from build123d import *

# Parameters (mm, degrees)
SKETCH1_R               = 19.05
BASE_EXTRUDE_DEPTH      = 47.625
CUT_EXTRUDE1_DEPTH      = 20.05
CUT_EXTRUDE1_DEPTH_BACK = 20.05
SKETCH8_W               = 20.32
SKETCH8_H               = 36.600526062
CUT_EXTRUDE5_DEPTH      = 47.625
CUT_EXTRUDE5_DEPTH_BACK = 20.0500001
SKETCH11_R              = 4.7625
CUT_EXTRUDE6_DEPTH      = 20.0500001
CUT_EXTRUDE6_DEPTH_BACK = 20.0500001
SKETCH12_R              = 6.35
BOSS_EXTRUDE1_DEPTH     = 19.05
CHAMFER3_SIZE           = 1.27
CHAMFER3_SIZE2          = 2.199704526
CUT_EXTRUDE7_DEPTH      = 12.7


with BuildPart() as part:
    # Sketch1 → Base-Extrude (new body)
    with BuildSketch(Plane(origin=(0, 0, 0), x_dir=(-1, 0, 0), z_dir=(0, 1, 0))):
        Circle(SKETCH1_R)
    extrude(amount=BASE_EXTRUDE_DEPTH)

    # Sketch2 → Cut-Extrude1 (cut, two sides)
    with BuildSketch(Plane.XY) as cut_extrude1_sk:
        with BuildLine():
            Line((9.525, 9.525), (9.525, 19.685))
            ThreePointArc((9.525, 19.685), (12.314807909, 26.420192091), (19.05, 29.21))
            Line((19.05, 29.21), (19.05, -1.366191125))
            Line((19.05, -1.366191125), (-19.05, -1.366191125))
            Line((-19.05, -1.366191125), (-19.05, 29.21))
            ThreePointArc((-19.05, 29.21), (-12.314807909, 26.420192091), (-9.525, 19.685))
            Line((-9.525, 19.685), (-9.525, 9.525))
            ThreePointArc((-9.525, 9.525), (0, 0), (9.525, 9.525))
        make_face()
    extrude(amount=CUT_EXTRUDE1_DEPTH, mode=Mode.SUBTRACT)
    extrude(cut_extrude1_sk.sketch, amount=-CUT_EXTRUDE1_DEPTH_BACK, mode=Mode.SUBTRACT)

    # Sketch8 → Cut-Extrude5 (cut, two sides)
    with BuildSketch(Plane(origin=(0, 0, 0), x_dir=(0, 0, -1), z_dir=(1, 0, 0))) as cut_extrude5_sk:
        with Locations((0, 10.844975795)):
            Rectangle(SKETCH8_W, SKETCH8_H)
    extrude(amount=CUT_EXTRUDE5_DEPTH, mode=Mode.SUBTRACT)
    extrude(cut_extrude5_sk.sketch, amount=-CUT_EXTRUDE5_DEPTH_BACK, mode=Mode.SUBTRACT)

    # Sketch11 → Cut-Extrude6 (cut, two sides)
    with BuildSketch(Plane.XY) as cut_extrude6_sk:
        with Locations((0, 9.525)):
            Circle(SKETCH11_R)
    extrude(amount=CUT_EXTRUDE6_DEPTH, mode=Mode.SUBTRACT)
    extrude(cut_extrude6_sk.sketch, amount=-CUT_EXTRUDE6_DEPTH_BACK, mode=Mode.SUBTRACT)

    # Sketch12 → Boss-Extrude1 (add)
    with BuildSketch(Plane(origin=(0, 47.625, 0), x_dir=(-1, 0, 0), z_dir=(0, 1, 0))):
        Circle(SKETCH12_R)
    extrude(amount=BOSS_EXTRUDE1_DEPTH)

    # Chamfer3
    chamfer3_edges = [part.edges().sort_by_distance(p)[0] for p in [
        (6.35, 66.675, 0),
    ]]
    chamfer3_side = [part.faces().sort_by_distance(p)[0] for p in [
        (6.35, 57.15, 0),
    ]]
    chamfer(chamfer3_edges, length=CHAMFER3_SIZE, length2=CHAMFER3_SIZE2, reference=chamfer3_side[0])

    # Sketch13 → Cut-Extrude7 (cut)
    with BuildSketch(Plane(origin=(0, 66.675, 0), x_dir=(-1, 0, 0), z_dir=(0, 1, 0))):
        with BuildLine():
            Line((-4.7625, 4.200130206), (-4.7625, -4.200130206))
            ThreePointArc((-4.7625, -4.200130206), (-6.35, 0), (-4.7625, 4.200130206))
        make_face()
    extrude(amount=-CUT_EXTRUDE7_DEPTH, mode=Mode.SUBTRACT)


solid = part.part
Here's how the part is built. I have some questions about the finished solid (model axes, mm). A direction names the side the tool comes from. Coordinates: 2 decimals unless noted, no trailing zeros. Order: outer loops, then holes, each group sorted by start corner. A loop starts at its lowest first (then second) coordinate and runs counter-clockwise, first axis right, second up. Notation, with made-up numbers: (33, -13) - (77, -13) arc R22 cw to (77, 1) - close; hole circle Ø7 at (75, 88). An arc over 180 degrees is marked (long way). Use CSV: the item, a comma, the result in double quotes. Start each with the question number.
1. For faces 1 (the face through (0, 29.145, 0)), 2 (the face through (-9.525, 15, 13)), 3 (the face through (4.762, 60, 0)), 4 (the face through (9.525, 15, 13)), 5 (the face through (5, 47.625, 5)), which set-ups out of +Z, -Z, +X, -X, +Y, -Y let a thin tool reach every point of the face, with its end or its side?
2. Please list where these lines run through material, in increasing order: line 1 (Y direction, x = 0, z = -13.75) (1 decimal); line 2 (Z direction, x = 0.5, y = 29); line 3 (Y direction, x = -15, z = -6.5) (3 decimals). Write a range as from..to.
3. I'm going to push flat-ended pins straight in: pin 1 (1.9 mm diameter, centred on y = 15, z = 13.5, fed in from +X) (3 decimals); pin 2 (1.9 mm diameter, centred on y = 17, z = -14.5, fed in from -X) (3 decimals); pin 3 (4 mm diameter, centred on x = 4.5, y = 16.5, fed in from -Z). Where does each tip first touch, or does it pass through?
4. Suppose I cut it at A-A on x = 0. Give the number of separate pieces and of enclosed holes in the cut face, then the cut area to 3 significant figures.
5. Suppose I cut it at D-D on y = 28. List the corners of the cut face in (x, z) for me.
6. If we mould it in two halves opening along X, with no side actions, what happens to faces 6 (the face through (-1.032, 4.876, 14.552)), 7 (the face through (0, 0, -14)), 8 (the face through (-1.032, 4.876, -14.552)), 9 (the face through (0, 18, -10.16))? For each: +X half, -X half, draft (parallel to the pull), parting line (faces both ways), or undercut.
Output:
1,face 1,"+X, -X, -Y"
1,face 2,"+Z, -Z, -X, -Y"
1,face 3,"+Z, -Z, +X, +Y"
1,face 4,"+Z, -Z, +X, -Y"
1,face 5,"+Y"
2,line 1,"y = 0..4.8, 14.3..47.6"
2,line 2,"z = -19.04..-10.16, 10.16..19.04"
2,line 3,"y = 29.145..47.625"
3,pin 1,"stops at x = 9.525"
3,pin 2,"stops at x = -9.525"
3,pin 3,"stops at z = -18.89"
4,separate pieces,"3"
4,enclosed holes,"0"
4,area,"1,290 mm2"
5,outline,"(-14.4, -12.47) arc R19.05 ccw to (14.4, -12.47) - (14.4, -10.16) - (-14.4, -10.16) - close; (-14.4, 10.16) - (14.4, 10.16) - (14.4, 12.47) arc R19.05 ccw to (-14.4, 12.47) - close"
6,face 6,"undercut"
6,face 7,"parting line"
6,face 8,"undercut"
6,face 9,"draft"
